Model file for the job. Use its own axes, mm. A direction names the side the tool comes from. Coordinates: 2 decimals unless noted, no trailing zeros. Write each loop counter-clockwise with the first axis right and the second up, starting at its lowest first coordinate (ties: lowest second). Pieces come first, ordered by that corner, then holes.
Q1. Band-saw the part on D-D, the plane y = 6.5. Write the cut outline in (x, z), plus the area to 3 significant figures.
Q2. Drill centre lines: probe 1 along Z at (x, y) = (-4.75, 6); probe 2 along X at (y, z) = (5.75, -1.25); probe 3 along X at (y, z) = (1, -1.75). Where is each one in solid material? Low to high.
Q3. Band-saw the part on B-B, the plane x = 0. Write the cut outline in (y, z).
Q4. Pin check, flat tips, straight feed: P1, Ø3, axis at x = -2.5, z = -1.5, coming from the -Y side; P2, Ø1.5, axis at y = 3.5, z = 0, coming from the +X side; P3, Ø4, axis at x = -3, z = -2, coming from the -Y side. Stop position of each tip, or through.
Q5. Band-saw the part on A-A, the plane y = 3.25. Write the cut outline in (x, z).
Q6. Band-saw the part on C-C, the plane z = -1.5. Write the cut outline in (x, y), plus the area to 3 significant figures.
Q7. Which spindle directions (+Z, -Z, +X, -X, +Y, -Y) get a long thin tool onto all of the face, cutting with end or side? Do faces 1 (the cylindrical face through (-0.16, 7.5, -2.27)), 2 (the cylindrical face through (7.506, 2.122, -0.01)). Say none if no direction does.
Q8. Pull direction Y, two halves, no side cores. Call faces 3 (the flat face through (1, 8, 3.75)), 4 (the cylindrical face through (-5.99, 5.53, -0.3)), 5 (the flat face through (8, 0, 0)): released by +Y, released by -Y, zero draft, split by the parting line, or undercut.
from build123d import *

# Parameters (mm, degrees)
CIRPATTERN1_COUNT = 4
CIRPATTERN1_ANGLE = 108


with BuildPart() as part:
    # Sweep1: sweep along a path in Sketch1
    with BuildLine(Plane.XY) as sweep1_path:
        ThreePointArc((-8.5, 0), (0, 8.5), (8.5, 0))
    # Sketch2 → Sweep1 (sweep)
    with BuildSketch(Plane(origin=(0, 0, 0), x_dir=(1, 0, 0), z_dir=(0, 1, 0))):
        Polygon((-7.5, -3.75), (-7.5, -0.75), (-7.8, -0.75), (-7.8, 0.75), (-7.5, 0.75), (-7.5, 3.75), (-8.5, 3.75), (-8.5, -3.75), align=None)
    sweep(path=sweep1_path.line)

    # Sketch3 → Cut-Revolve1 (revolve, cut)
    with BuildSketch(Plane.XY):
        Polygon((4.938511893, 3.588038915), (15.375889989, 11.171237983), (15.963675241, 10.362220989), (5.526297145, 2.779021921), align=None)
    cut_revolve1 = revolve(axis=Axis((4.938511893, 3.588038915, 0), (0.8090169943749489, 0.5877852522924712, 0)), mode=Mode.SUBTRACT)

    # CirPattern1: Cut-Revolve1 ×4 about axis
    cirpattern1_axis = Axis((0, 0, -11.55), (0, 0, 1))
    for i in range(1, CIRPATTERN1_COUNT):
        add(cut_revolve1.rotate(cirpattern1_axis, i * CIRPATTERN1_ANGLE / (CIRPATTERN1_COUNT - 1)), mode=Mode.SUBTRACT)


solid = part.part
Answer sheet:
1. outline: (-5.48, -3.75) - (-3.74, -3.75) - (-3.74, -0.75) - (-4.31, -0.75) - (-4.31, 0.75) - (-3.74, 0.75) - (-3.74, 3.75) - (-5.48, 3.75) - close; (3.74, -3.75) - (5.48, -3.75) - (5.48, 3.75) - (3.74, 3.75) - (3.74, 0.75) - (4.31, 0.75) - (4.31, -0.75) - (3.74, -0.75) - close
1. area: 24.3 mm2
2. probe 1: z = -3.75 to -0.75, 0.75 to 3.75
2. probe 2: x = -6.26 to -4.82, 4.82 to 6.26
2. probe 3: x = -8.44 to -7.43, 7.43 to 8.44
3. outline: (7.5, -3.75) - (8.5, -3.75) - (8.5, 3.75) - (7.5, 3.75) - (7.5, 0.75) - (7.8, 0.75) - (7.8, -0.75) - (7.5, -0.75) - close
4. P1: stops at y = 6.34
4. P2: stops at x = 8.04
4. P3: stops at y = 5.59
5. outline: (-7.85, -3.75) - (-6.76, -3.75) - (-6.76, -0.75) - (-7.09, -0.75) - (-7.09, 0.75) - (-6.76, 0.75) - (-6.76, 3.75) - (-7.85, 3.75) - close; (6.76, -3.75) - (7.85, -3.75) - (7.85, 3.75) - (6.76, 3.75) - (6.76, 0.75) - (7.09, 0.75) - (7.09, -0.75) - (6.76, -0.75) - close
6. outline: (-8.5, 0) - (-7.5, 0) arc R7.5 cw to (7.5, 0) - (8.5, 0) arc R8.5 ccw to start
6. area: 25.1 mm2
7. face 1: +Z, -Z, -Y
7. face 2: -Y
8. face 3: zero draft
8. face 4: undercut
8. face 5: released by -Y
